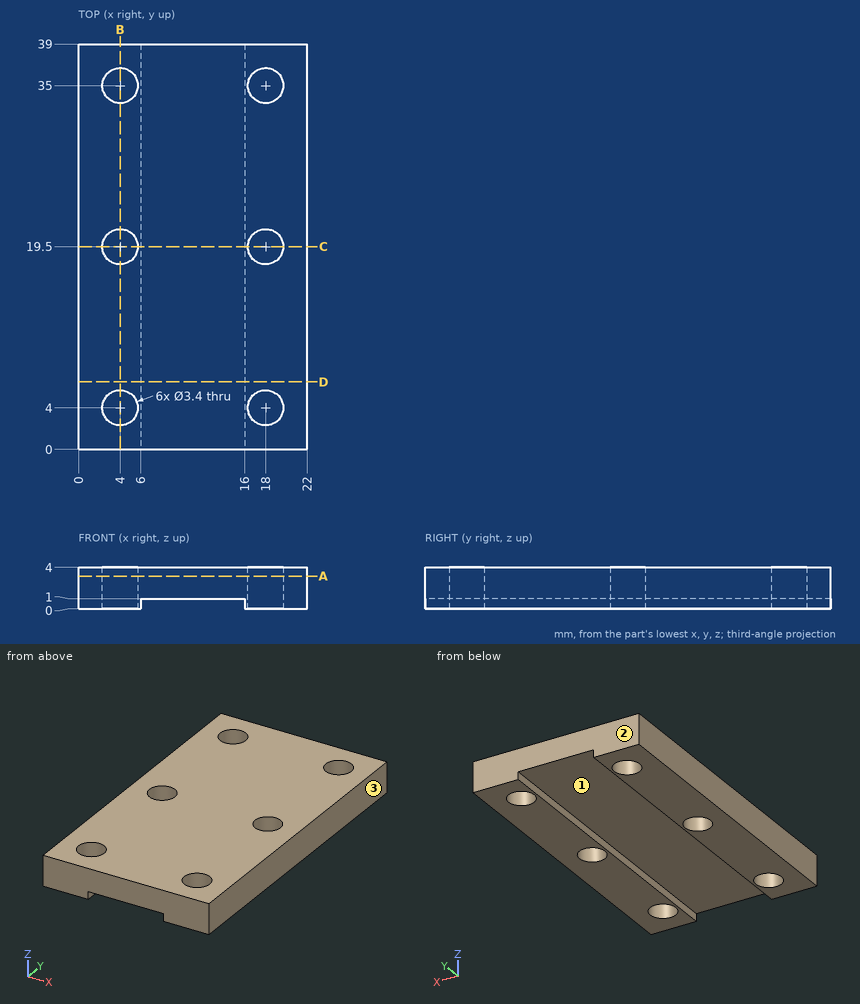
Print and shaded views of the part. All mm, measured from the part's lowest x, y and z. Give positions to 0.01 mm unless a question says otherwise; leave off trailing zeros. Loops run counter-clockwise (first coordinate to the right, second up) from the corner with the lowest first, then second, coordinate; pieces in that order, holes last. Notation, with made-up numbers: M 83,-18.5 L 89,-18.5 A17 ccw 89,10.5 Z; hole C 81.25,75.25 d10. An arc over 180 degrees is marked long. Write each question's results on one line, items separated by ' | '.
Q1. Band-saw the part on D-D on y = 6.5. Write the cut outline in (x, z).
Geometry check:
outline: M 0,0 L 6,0 L 6,1 L 16,1 L 16,0 L 22,0 L 22,4 L 0,4 Z
Q2. Probe probe 1 along Y at (x, z) = (4, 2.15); probe 2 along X at (y, z) = (16.5, 0.3); probe 3 along X at (y, z) = (36, 0.65). List the from-to ranges inside material, lowest first.
Geometry check:
probe 1: y = 0 to 2.3, 5.7 to 17.8, 21.2 to 33.3, 36.7 to 39 | probe 2: x = 0 to 6, 16 to 22 | probe 3: x = 0 to 2.63, 5.37 to 6, 16 to 16.63, 19.37 to 22
Q3. Mould opens along X. For the marked faces 1, 2 and 3 say: pulls with the +X half, pulls with the -X half, needs draft (parallel to the pull), parting line crosses it, or undercut.
Geometry check:
face 1: undercut | face 2: needs draft | face 3: pulls with the +X half
Q4. Flat gauge pin, fed straight in: P1, Ø2, axis at x = 4, y = 19.5, coming from the -Z side. Where does the tip first touch, or does it go through?
Geometry check:
P1: passes through
Q5. Band-saw the part on C-C on y = 19.5. Write the cut outline in (x, z), and give its area (3 significant figures).
Geometry check:
outline: M 0,0 L 2.3,0 L 2.3,4 L 0,4 Z; M 5.7,0 L 6,0 L 6,1 L 16,1 L 16,0 L 16.3,0 L 16.3,4 L 5.7,4 Z; M 19.7,0 L 22,0 L 22,4 L 19.7,4 Z | area: 50.8 mm²
Q6. Band-saw the part on B-B on x = 4. Write the cut outline in (y, z).
Geometry check:
outline: M 0,0 L 2.3,0 L 2.3,4 L 0,4 Z; M 5.7,0 L 17.8,0 L 17.8,4 L 5.7,4 Z; M 21.2,0 L 33.3,0 L 33.3,4 L 21.2,4 Z; M 36.7,0 L 39,0 L 39,4 L 36.7,4 Z
Q7. Band-saw the part on A-A on z = 3.15. Write the cut outline in (x, y).
Geometry check:
outline: M 0,0 L 22,0 L 22,39 L 0,39 Z; hole C 4,4 d3.4; hole C 4,19.5 d3.4; hole C 4,35 d3.4; hole C 18,4 d3.4; hole C 18,19.5 d3.4; hole C 18,35 d3.4
